Design review of the part built by this model. Coordinates are the model's own, in mm. Face numbers are marked on the shaded views. Round coordinates to 2 decimals unless told otherwise and drop trailing zeros. Write each loop counter-clockwise with the first axis right and the second up, starting at its lowest first coordinate (ties: lowest second). Pieces come first, ordered by that corner, then holes. Notation, with made-up numbers: M 44,69.5 L 88,69.5 A29 cw 88,108.5 Z; hole C 64.5,47 d6. An arc over 180 degrees is marked long. One line per question, with ' | ' between items. Start each with the question number.
Item 1: Add section C-C, the plane z = 1.1. State the section outline as (x, y) points, and give its area (3 significant figures).
Item 2: Insertion check: pin 1 Ø1.5 at (y, z) = (5, 4) entering from +X; pin 2 Ø1 at (y, z) = (2.5, 3) entering from +X; pin 3 Ø13.5 at (x, y) = (0, 0) entering from +Z. Each pin has a flat end and moves straight along its axis. Give the tip position at first contact, or say it passes through.
Item 3: Draft analysis for pull direction X (two halves, no side actions). For the marked faces 1, 2 and 3, state which applies: released by +X, released by -X, zero draft, split by the parting line, or undercut.
Item 4: For L1, parallel to Y at x = 0, z = 2.5; L2, parallel to Y at x = 0, z = 4.05; L3, parallel to X at y = -1.25, z = 3, list the stretches that pass through material, from the lowest coordinate up.
Item 5: Add section A-A, the plane y = 0. State the section outline as (x, z) points, and give its area (3 significant figures).
```python
from build123d import *

# Parameters (mm, degrees)
SKETCH_1_R      = 13
SKETCH_1_R_2    = 8.5
EXTRUDE_1_DEPTH = 5
SKETCH_2_R      = 14
SKETCH_2_R_2    = 13
EXTRUDE_2_DEPTH = 1
FILLET_1_R      = 0.3


with BuildPart() as part:
    # 草图1 → 凸台-拉伸1 (new body)
    with BuildSketch(Plane.XY):
        Circle(SKETCH_1_R)
        Circle(SKETCH_1_R_2, mode=Mode.SUBTRACT)
    extrude(amount=EXTRUDE_1_DEPTH)

    # 草图2 → 凸台-拉伸2 (add)
    with BuildSketch(Plane.XY.offset(5)):
        Circle(SKETCH_2_R)
        Circle(SKETCH_2_R_2, mode=Mode.SUBTRACT)
    extrude(amount=-EXTRUDE_2_DEPTH)

    # 圆角1
    fillet_1_edges = [part.edges().sort_by_distance(p)[0] for p in [
        (-13, 0, 0),
    ]]
    fillet(fillet_1_edges, radius=FILLET_1_R)


solid = part.part
```
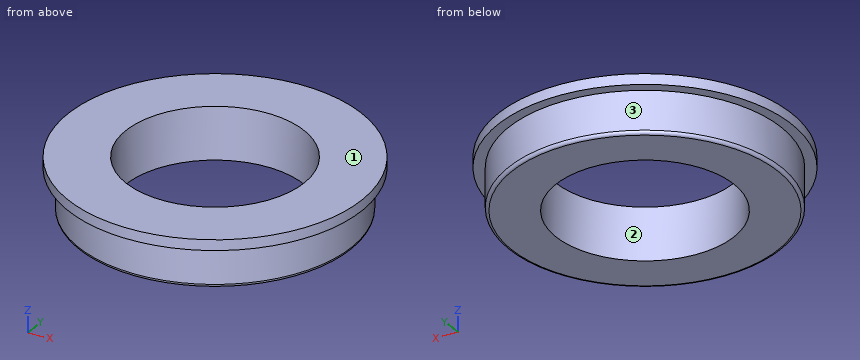
Computed values:
1) outline: C 0,0 d26; hole C 0,0 d17 | area: 304 mm^2
2) pin 1: stops at x = 13.34 | pin 2: stops at x = 12.85 | pin 3: passes through
3) face 1: zero draft | face 2: undercut | face 3: split by the parting line
4) L1: y = -13 to -8.5, 8.5 to 13 | L2: y = -14 to -8.5, 8.5 to 14 | L3: x = -12.94 to -8.41, 8.41 to 12.94
5) outline: M -14,4 L -13,4 L -13,0.3 A0.3 ccw -12.7,0 L -8.5,0 L -8.5,5 L -14,5 Z; M 8.5,0 L 12.7,0 A0.3 ccw 13,0.3 L 13,4 L 14,4 L 14,5 L 8.5,5 Z | area: 47.0 mm^2
